Design review of the part built by this model. Coordinates are the model's own, in mm. Coordinates: 2 decimals unless noted, no trailing zeros. Write each loop counter-clockwise with the first axis right and the second up, starting at its lowest first coordinate (ties: lowest second). Pieces come first, ordered by that corner, then holes. Notation, with made-up numbers: (-29.75, 37) - (16.25, 37) arc R32 ccw to (16.25, 63) - close; hole circle Ø4 at (5, 74). An arc over 180 degrees is marked (long way). Answer as a JSON object with one key per item and string values.
```python
from build123d import *

# Parameters (mm, degrees)
BOSS_EXTRUDE1_DEPTH = 5
SKETCH3_R           = 5
BOSS_EXTRUDE2_DEPTH = 5
SKETCH4_R           = 1.5
BOSS_EXTRUDE3_DEPTH = 8


with BuildPart() as part:
    # Sketch1 → Boss-Extrude1 (new body)
    with BuildSketch(Plane.XY):
        with BuildLine():
            Line((-107.5, 7.5), (107.5, 7.5))
            Line((107.5, 7.5), (107.5, 117.5))
            ThreePointArc((107.5, 117.5), (117.5, 127.5), (127.5, 117.5))
            Line((127.5, 117.5), (127.5, -117.5))
            ThreePointArc((127.5, -117.5), (117.5, -127.5), (107.5, -117.5))
            Line((107.5, -117.5), (107.5, -7.5))
            Line((107.5, -7.5), (-107.5, -7.5))
            Line((-107.5, -7.5), (-107.5, -117.5))
            ThreePointArc((-107.5, -117.5), (-117.5, -127.5), (-127.5, -117.5))
            Line((-127.5, -117.5), (-127.5, 117.5))
            ThreePointArc((-127.5, 117.5), (-117.5, 127.5), (-107.5, 117.5))
            Line((-107.5, 117.5), (-107.5, 7.5))
        make_face()
    extrude(amount=BOSS_EXTRUDE1_DEPTH)

    # Sketch3 → Boss-Extrude2 (add)
    with BuildSketch(Plane.XY.offset(5)):
        with Locations((117.5, -117.5)):
            Circle(SKETCH3_R)
        with Locations((117.5, 117.5)):
            Circle(SKETCH3_R)
        with Locations((-117.5, 117.5)):
            Circle(SKETCH3_R)
        with Locations((-117.5, -117.5)):
            Circle(SKETCH3_R)
    extrude(amount=BOSS_EXTRUDE2_DEPTH)

    # Sketch4 → Boss-Extrude3 (add)
    with BuildSketch(Plane.XY.offset(10)):
        with Locations((-117.5, 117.5)):
            Circle(SKETCH4_R)
        with Locations((-117.5, -117.5)):
            Circle(SKETCH4_R)
        with Locations((117.5, -117.5)):
            Circle(SKETCH4_R)
        with Locations((117.5, 117.5)):
            Circle(SKETCH4_R)
    extrude(amount=BOSS_EXTRUDE3_DEPTH)


solid = part.part
```
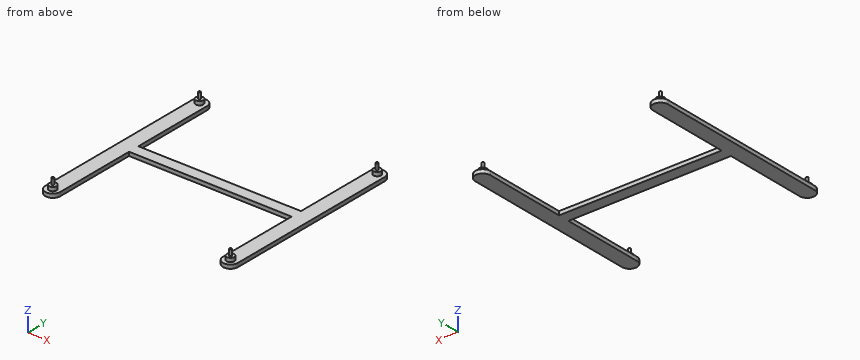
(1) For pin 1 (2.5 mm diameter, centred on x = 7.5, z = 2, fed in from +Y); pin 2 (5.5 mm diameter, centred on x = 48, z = 3, fed in from -Y); pin 3 (8 mm diameter, centred on y = -44, z = 12, fed in from -X), all flat-tipped, find the tip position at first contact; note any pin that passes through.
Solved:
{"pin 1": "stops at y = 7.5", "pin 2": "stops at y = -7.5", "pin 3": "passes through"}
(2) To check wall thickness, follow line 1 (X direction, y = 26.5, z = 2.5); line 2 (Y direction, x = -44, z = 3); line 3 (Z direction, x = 112, y = 8). State the ranges of each line that lie inside material, in increasing order. Write a range as from..to.
Solved:
{"line 1": "x = -127.5..-107.5, 107.5..127.5", "line 2": "y = -7.5..7.5", "line 3": "z = 0..5"}
(3) Take a section at A-A, the plane y = 86. Write out the cut boundary in (x, z), and give its area (3 significant figures).
Solved:
{"outline": "(-127.5, 0) - (-107.5, 0) - (-107.5, 5) - (-127.5, 5) - close; (107.5, 0) - (127.5, 0) - (127.5, 5) - (107.5, 5) - close", "area": "200 mm^2"}
(4) Take a section at B-B, the plane x = -68. Write out the cut boundary in (y, z), and give its area (3 significant figures).
Solved:
{"outline": "(-7.5, 0) - (7.5, 0) - (7.5, 5) - (-7.5, 5) - close", "area": "75.0 mm^2"}
